```python
from build123d import *

# Parameters (mm, degrees)
SKETCH1_R           = 9
SKETCH1_R_2         = 7.5
BOSS_EXTRUDE1_DEPTH = 18
SKETCH2_R           = 7.5
SKETCH2_R_2         = 3
BOSS_EXTRUDE2_DEPTH = 4


with BuildPart() as part:
    # Sketch1 → Boss-Extrude1 (new body)
    with BuildSketch(Plane(origin=(0, 0, 0), x_dir=(1, 0, 0), z_dir=(0, 1, 0))):
        with Locations(Location((0, 0, 0), (0, 0, 270))):
            Circle(SKETCH1_R)
        with Locations(Location((0, 0, 0), (0, 0, 270))):
            Circle(SKETCH1_R_2, mode=Mode.SUBTRACT)
    extrude(amount=BOSS_EXTRUDE1_DEPTH)

    # Sketch2 → Boss-Extrude2 (add, symmetric)
    with BuildSketch(Plane(origin=(0, 9, 0), x_dir=(1, 0, 0), z_dir=(0, 1, 0))):
        with Locations(Location((0, 0, 0), (0, 0, 270))):
            Circle(SKETCH2_R)
        with Locations(Location((0, 0, 0), (0, 0, 270))):
            Circle(SKETCH2_R_2, mode=Mode.SUBTRACT)
    extrude(amount=BOSS_EXTRUDE2_DEPTH, both=True)


solid = part.part
```
Can you work these out from the model? Positions are in its coordinate system, mm. A direction names the side the tool comes from. Coordinates: 2 decimals unless noted, no trailing zeros. Order: outer loops, then holes, each group sorted by start corner. A loop starts at its lowest first (then second) coordinate and runs counter-clockwise, first axis right, second up.
1. Thinking about a two-plate mould opening in X: for faces 4 (the face through (2.703, 8.874, 8.584)), 5 (the face through (0.1, 13, 3.2)), 6 (the face through (7.4, 0, -2)), which applies, +X half, -X half, draft (parallel to the pull), parting line (faces both ways), or undercut?
2. If we section it at D-D (z = 6.5): Please give me the cut outline in (x, y).
3. For faces 1 (the face through (7.4, 18, -2)), 2 (the face through (0.33, 15.465, -7.493)), 3 (the face through (0.1, 5, 3.2)), which set-ups out of +Z, -Z, +X, -X, +Y, -Y let a thin tool reach every point of the face, with its end or its side?
4. I need wall thicknesses on line 1 (X direction, y = 2.6, z = 0); line 2 (Y direction, x = 3.75, z = 2.5); line 3 (X direction, y = 11.25, z = 0). Which ranges of each line are inside material? Lowest first, please.
5. If we section it at A-A (z = 0): Please give me the cut outline in (x, y), then the cut area to 3 significant figures.
6. I'm going to push flat-ended pins straight in: pin 1 (8 mm diameter, centred on x = -6, y = 2, fed in from +Z); pin 2 (1.5 mm diameter, centred on x = 4, z = -5, fed in from -Y); pin 3 (8 mm diameter, centred on y = 7, z = 5.5, fed in from +X). Where does each tip first touch, or does it pass through?
7. If we section it at B-B (x = 0): Please give me the cut outline in (y, z).
8. If we section it at C-C (y = 9.5): Please give me the cut outline in (x, z), then the cut area to 3 significant figures.
Entries:
1. face 4: parting line
1. face 5: undercut
1. face 6: draft
2. outline: (-6.22, 0) - (-3.74, 0) - (-3.74, 5) - (3.74, 5) - (3.74, 0) - (6.22, 0) - (6.22, 18) - (3.74, 18) - (3.74, 13) - (-3.74, 13) - (-3.74, 18) - (-6.22, 18) - close
3. face 1: +Z, -Z, +X, -X, +Y
3. face 2: +Y
3. face 3: -Y
4. line 1: x = -9 to -7.5, 7.5 to 9
4. line 2: y = 5 to 13
4. line 3: x = -9 to -3, 3 to 9
5. outline: (-9, 0) - (-7.5, 0) - (-7.5, 5) - (-3, 5) - (-3, 13) - (-7.5, 13) - (-7.5, 18) - (-9, 18) - close; (3, 5) - (7.5, 5) - (7.5, 0) - (9, 0) - (9, 18) - (7.5, 18) - (7.5, 13) - (3, 13) - close
5. area: 126 mm2
6. pin 1: stops at z = 8.77
6. pin 2: stops at y = 5
6. pin 3: stops at x = 8.87
7. outline: (0, -9) - (18, -9) - (18, -7.5) - (13, -7.5) - (13, -3) - (5, -3) - (5, -7.5) - (0, -7.5) - close; (0, 7.5) - (5, 7.5) - (5, 3) - (13, 3) - (13, 7.5) - (18, 7.5) - (18, 9) - (0, 9) - close
8. outline: circle Ø18 at (0, 0); hole circle Ø6 at (0, 0)
8. area: 226 mm2
